from build123d import *

# Parameters (mm, degrees)
SKETCH1_R           = 8.001
BOSS_EXTRUDE1_DEPTH = 3.048
BOSS_EXTRUDE2_DEPTH = 3.048
FILLET1_R           = 1.5748
FILLET2_R           = 4.6228


with BuildPart() as part:
    # Sketch1 → Boss-Extrude1 (new body)
    with BuildSketch(Plane.XY):
        with BuildLine():
            Line((-23.876, 6.35), (-12.804579401, 27.330865424))
            ThreePointArc((-12.804579401, 27.330865424), (0, 35.052), (12.804579401, 27.330865424))
            Line((12.804579401, 27.330865424), (23.876, 6.35))
            Line((23.876, 6.35), (23.876, 0))
            Line((23.876, 0), (-23.876, 0))
            Line((-23.876, 0), (-23.876, 6.35))
        make_face()
        with Locations((0, 20.574)):
            Circle(SKETCH1_R, mode=Mode.SUBTRACT)
    extrude(amount=-BOSS_EXTRUDE1_DEPTH)

    # Sketch2 → Boss-Extrude2 (add)
    with BuildSketch(Plane.XZ):
        with BuildLine():
            Line((23.876, -10.795), (19.05, -10.795))
            ThreePointArc((19.05, -10.795), (15.621, -14.224), (19.05, -17.653))
            Line((19.05, -17.653), (23.876, -17.653))
            Line((23.876, -17.653), (23.876, -22.817666667))
            ThreePointArc((23.876, -22.817666667), (23.119652078, -24.643652078), (21.293666667, -25.4))
            Line((21.293666667, -25.4), (-21.293666667, -25.4))
            ThreePointArc((-21.293666667, -25.4), (-23.119652078, -24.643652078), (-23.876, -22.817666667))
            Line((-23.876, -22.817666667), (-23.876, -17.653))
            Line((-23.876, -17.653), (-19.05, -17.653))
            ThreePointArc((-19.05, -17.653), (-15.621, -14.224), (-19.05, -10.795))
            Line((-19.05, -10.795), (-23.876, -10.795))
            Line((-23.876, -10.795), (-23.876, 0))
            Line((-23.876, 0), (23.876, 0))
            Line((23.876, 0), (23.876, -10.795))
        make_face()
    extrude(amount=-BOSS_EXTRUDE2_DEPTH)

    # Fillet1
    fillet1_edges = [part.edges().sort_by_distance(p)[0] for p in [
        (0, 3.048, -3.048),
    ]]
    fillet(fillet1_edges, radius=FILLET1_R)

    # Fillet2
    fillet2_edges = [part.edges().sort_by_distance(p)[0] for p in [
        (0, 0, 0),
    ]]
    fillet(fillet2_edges, radius=FILLET2_R)


solid = part.part
CAD build for the part. Positions are in the model's coordinates, mm. A direction names the side the tool comes from. Round coordinates to 2 decimals unless told otherwise and drop trailing zeros. Loops run counter-clockwise (first coordinate to the right, second up) from the corner with the lowest first, then second, coordinate; pieces in that order, holes last. Notation, with made-up numbers: M 42,31 L 69,31 A19 ccw 69,63 Z; hole C 32.25,13 d10. An arc over 180 degrees is marked long. One line per question, with ' | ' between items. Start each with the question number.
Item 1: Which spindle directions (+Z, -Z, +X, -X, +Y, -Y) get a long thin tool onto all of the face, cutting with end or side? Do faces 1 (the flat face through (0, 3.048, -15)), 2 (the flat face through (-21, 2, -10.795)), 3 (the cylindrical face through (-0.33, 1.39, -1.32)). Say none if no direction does.
Item 2: Cut at C-C, the plane x = -11. Write the cut outline in (y, z), plus the area to 3 significant figures.
Item 3: Cut at D-D, the plane z = -7.25. Write the cut outline in (x, y).
Item 4: Cut at B-B, the plane y = 24. Write the cut outline in (x, z).
Item 5: Cut at A-A, the plane x = 0. Write the cut outline in (y, z) (3 decimals).
Item 6: Pin check, flat tips, straight feed: pin 1 Ø4 at (x, y) = (-12, 9) entering from +Z; pin 2 Ø6 at (y, z) = (25, -5) entering from -X; pin 3 Ø2.5 at (x, y) = (21.5, 1) entering from +Z; pin 4 Ø0.9 at (x, y) = (-22, 1.5) entering from +Z. Stop position of each tip, or through.
Item 7: Two-plate mould, pull along Z, no slides. Class faces 4 (the flat face through (23.876, 2, -5)), 5 (the flat face through (-21, 2, -17.653)), 6 (the cylindrical face through (-23.099, 1.503, -24.664)): pulls with the +Z half, pulls with the -Z half, needs draft (parallel to the pull), parting line crosses it, or undercut.
Item 8: Wall check: line 1 (Y direction, x = -21, z = -22); line 2 (Y direction, x = 0, z = -1.3) (3 decimals); line 3 (Z direction, x = -9.5, y = 5). Give the ranges that are in metal, low to high.
Responses:
1) face 1: -Z, +X, -X, +Y | face 2: -X, +Y, -Y | face 3: +Z, +X, -X, -Y
2) outline: M 0,-25.4 L 3.05,-25.4 L 3.05,-4.62 A1.57 cw 4.62,-3.05 L 29.99,-3.05 L 29.99,0 L 4.62,0 A4.62 ccw 0,-4.62 Z | area: 155 mm²
3) outline: M -23.88,0 L 23.88,0 L 23.88,3.05 L -23.88,3.05 Z
4) outline: M -14.56,-3.05 L -7.23,-3.05 L -7.23,0 L -14.56,0 Z; M 7.23,-3.05 L 14.56,-3.05 L 14.56,0 L 7.23,0 Z
5) outline: M 0,-25.4 L 3.048,-25.4 L 3.048,-4.623 A1.575 cw 4.623,-3.048 L 12.573,-3.048 L 12.573,0 L 4.623,0 A4.623 ccw 0,-4.623 Z; M 28.575,-3.048 L 35.052,-3.048 L 35.052,0 L 28.575,0 Z
6) pin 1: stops at z = 0 | pin 2: stops at x = -15.24 | pin 3: stops at z = -0.66 | pin 4: stops at z = -0.85
7) face 4: needs draft | face 5: undercut | face 6: pulls with the -Z half
8) line 1: y = 0 to 3.05 | line 2: y = 1.409 to 12.573, 28.575 to 35.052 | line 3: z = -3.05 to 0
